Here's how the part is built. I have some questions about the finished solid (model axes, mm). Face numbers are marked on the shaded views. A direction names the side the tool comes from. Round coordinates to 2 decimals unless told otherwise and drop trailing zeros. Loops run counter-clockwise (first coordinate to the right, second up) from the corner with the lowest first, then second, coordinate; pieces in that order, holes last. Notation, with made-up numbers: (-24, 4) - (-18, 4) arc R34 cw to (-18, 38) - close; hole circle Ø4 at (42.5, 9.25). An arc over 180 degrees is marked (long way). Answer as a JSON object with one key per item and string values. Group by question number.
1) I want a section at C-C, the plane y = 7.75. Please give me the cut outline in (x, z), then the cut area to 3 significant figures.
2) I want a section at D-D, the plane z = 8. Please give me the cut outline in (x, y), then the cut area to 3 significant figures.
3) I want a section at B-B, the plane x = -3.5. Please give me the cut outline in (y, z).
4) Which directions (+Z, -Z, +X, -X, +Y, -Y) give clear straight access to the entire face, cutting with the end or side of a thin tool? Please do the marked faces 1, 2 and 3.
5) Will these pins go through, and if not, where does the flat tip stop? P1, Ø1.8, axis at x = 0, y = 0.5, coming from the +Z side; P2, Ø12, axis at y = -7, z = 26.5, coming from the +X side; P3, Ø0.9, axis at y = 7.5, z = 27, coming from the -X side.
6) If we mould it in two halves opening along Y, with no side actions, what happens to the marked faces 4, 5 and 6? For each: pulls with the +Y half, pulls with the -Y half, needs draft (parallel to the pull), parting line crosses it, or undercut.
7) If I drill on line 1 along Y through (x, z) = (0, 34.8); line 2 along Y through (x, z) = (0, 8); line 3 along Z through (x, y) = (2.25, -3.5), over which ranges is the centre line in solid material (lowest first)? Write a range as [from, to].
8) I want a section at A-A, the plane y = 0. Please give me the cut outline in (x, z), then the cut area to 3 significant figures.
from build123d import *
from build123d.topology import SkipClean

# Parameters (mm, degrees)
SKETCH_1_R           = 8.5
EXTRUDE_1_DEPTH      = 35
SKETCH_3_W           = 4
SKETCH_3_H           = 4
CUT_EXTRUDE_1_DEPTH  = 14
EXTRUDE_2_REACH      = 41.016
EXTRUDE_2_END_RADIUS = 8.5
EXTRUDE_3_REACH      = 41.016
EXTRUDE_3_END_RADIUS = 8.5
SKETCH_6_R           = 10
SKETCH_6_R_2         = 8.5
EXTRUDE_4_DEPTH      = 7
SKETCH_7_R           = 8.5
EXTRUDE_5_DEPTH      = 3
EXTRUDE_6_REACH      = 44.617
EXTRUDE_6_END_RADIUS = 8.5
CUT_EXTRUDE_2_DEPTH  = 43.617484675
FILLET_1_R           = 2
CUT_EXTRUDE_START    = -3
SKETCH_10_R          = 10
SKETCH_10_R_2        = 8.5
CUT_EXTRUDE_3_DEPTH  = 3
SKETCH_11_R          = 8.5
EXTRUDE_7_DEPTH      = 1
SKETCH_12_R          = 1
CUT_EXTRUDE_4_DEPTH  = 5
CUT_EXTRUDE_5_DEPTH  = 2
EXTRUDE_START        = 3
SKETCH_14_R          = 1
SKETCH_14_R_2        = 0.85
EXTRUDE_8_DEPTH      = 3
FILLET_2_R           = 0.2
SKETCH_15_W          = 8
SKETCH_15_H          = 8
CUT_EXTRUDE_6_DEPTH  = 6


with BuildPart() as part:
    # 草图1 → 凸台-拉伸1 (new body)
    with BuildSketch(Plane.XY):
        Circle(SKETCH_1_R)
    extrude(amount=EXTRUDE_1_DEPTH)

    # 草图3 → 切除-拉伸1 (cut)
    with BuildSketch(Plane.XY.offset(35)):
        with Locations((0, 8.5)):
            Rectangle(SKETCH_3_W, SKETCH_3_H)
    extrude(amount=-CUT_EXTRUDE_1_DEPTH, mode=Mode.SUBTRACT)

    # 凸台-拉伸2: up to this cylinder (the profile starts inside it)
    with SkipClean():  # the faces are left unmerged after this step: merging them gives an invalid solid
        extrude_2_end = Plane(origin=(0, 0, 21.446736), z_dir=(0, 0, -1)) * Cylinder(EXTRUDE_2_END_RADIUS, 100.032, mode=Mode.PRIVATE)
        # 草图4 → 凸台-拉伸2 (add, up to the surface)
        with BuildSketch(Plane(origin=(0, 6.5, 0), x_dir=(1, 0, 0), z_dir=(0, 1, 0)), mode=Mode.PRIVATE) as extrude_2_sk1:
            with BuildLine():
                Line((2, -21), (0, -21))
                ThreePointArc((0, -21), (1.414213562, -21.585786438), (2, -23))
                Line((2, -23), (2, -21))
            make_face()
        extrude_2_tool1 = extrude(extrude_2_sk1.sketch, amount=EXTRUDE_2_REACH, mode=Mode.PRIVATE) & extrude_2_end
        add(extrude_2_tool1.solids().sort_by_distance((1.553264, 6.5, 21.446736))[0])
        # 草图4 → 凸台-拉伸2 (add, up to the surface)
        with BuildSketch(Plane(origin=(0, 6.5, 0), x_dir=(1, 0, 0), z_dir=(0, 1, 0)), mode=Mode.PRIVATE) as extrude_2_sk2:
            with BuildLine():
                Line((-2, -21), (-2, -23))
                ThreePointArc((-2, -23), (-1.414213562, -21.585786438), (0, -21))
                Line((0, -21), (-2, -21))
            make_face()
        extrude_2_tool2 = extrude(extrude_2_sk2.sketch, amount=EXTRUDE_2_REACH, mode=Mode.PRIVATE) & extrude_2_end
        add(extrude_2_tool2.solids().sort_by_distance((-1.553264, 6.5, 21.446736))[0])

    # 凸台-拉伸3: up to this cylinder (the profile starts inside it)
    with SkipClean():  # the faces are left unmerged after this step: merging them gives an invalid solid
        extrude_3_end = Plane(origin=(0, 0, 32.762904), z_dir=(0, 0, -1)) * Cylinder(EXTRUDE_3_END_RADIUS, 100.032, mode=Mode.PRIVATE)
        # 草图5 → 凸台-拉伸3 (add, up to the surface)
        with BuildSketch(Plane(origin=(0, 6.5, 0), x_dir=(1, 0, 0), z_dir=(0, 1, 0)), mode=Mode.PRIVATE) as extrude_3_sk1:
            with BuildLine():
                Line((-2, -29), (-2, -35))
                Line((-2, -35), (2, -35))
                Line((2, -35), (2, -29))
                ThreePointArc((2, -29), (0, -31), (-2, -29))
            make_face()
        extrude_3_tool1 = extrude(extrude_3_sk1.sketch, amount=EXTRUDE_3_REACH, mode=Mode.PRIVATE) & extrude_3_end
        add(extrude_3_tool1.solids().sort_by_distance((0, 6.5, 32.762904))[0])

    # 草图6 → 凸台-拉伸4 (add)
    with BuildSketch(Plane(origin=(0, 0, 0), x_dir=(-1, 0, 0), z_dir=(0, 0, -1))):
        Circle(SKETCH_6_R)
        Circle(SKETCH_6_R_2, mode=Mode.SUBTRACT)
    extrude(amount=-EXTRUDE_4_DEPTH)

    # 草图7 → 凸台-拉伸5 (add)
    with SkipClean():  # the faces are left unmerged after this step: merging them gives an invalid solid
        with BuildSketch(Plane.XY.offset(35)):
            with Locations(Location((0, 0, 0), (0, 0, 180))):
                Circle(SKETCH_7_R)
        extrude(amount=EXTRUDE_5_DEPTH)

    # 凸台-拉伸6: up to this cylinder (the profile starts inside it)
    with SkipClean():  # the faces are left unmerged after this step: merging them gives an invalid solid
        extrude_6_end = Plane(origin=(0, 0, 22.258337), z_dir=(0, 0, -1)) * Cylinder(EXTRUDE_6_END_RADIUS, 107.234, mode=Mode.PRIVATE)
        # 草图8 → 凸台-拉伸6 (add, up to the surface)
        with BuildSketch(Plane(origin=(0, 6.5, 0), x_dir=(1, 0, 0), z_dir=(0, 1, 0)), mode=Mode.PRIVATE) as extrude_6_sk1:
            with BuildLine():
                Line((-2, -23), (-2, -23.2))
                Line((-2, -23.2), (2, -23.2))
                Line((2, -23.2), (2, -23))
                ThreePointArc((2, -23), (0, -21), (-2, -23))
            make_face()
        extrude_6_tool1 = extrude(extrude_6_sk1.sketch, amount=EXTRUDE_6_REACH, mode=Mode.PRIVATE) & extrude_6_end
        add(extrude_6_tool1.solids().sort_by_distance((0, 6.5, 22.258337))[0])

    # 草图9 → 切除-拉伸2 (cut, through all)
    with SkipClean():  # the faces are left unmerged after this step: merging them gives an invalid solid
        with BuildSketch(Plane(origin=(0, 6.5, 0), x_dir=(1, 0, 0), z_dir=(0, 1, 0))):
            with BuildLine():
                Line((-2, -29), (-2, -29.5))
                Line((-2, -29.5), (-2, -31.5))
                ThreePointArc((-2, -31.5), (0, -33.5), (2, -31.5))
                Line((2, -31.5), (2, -29.5))
                Line((2, -29.5), (2, -29))
                Line((2, -29), (-2, -29))
            make_face()
        extrude(amount=CUT_EXTRUDE_2_DEPTH, mode=Mode.SUBTRACT)

    # 圆角1
    # the kernel refuses this fillet: 2 mm, written as the material it adds along each edge
    with BuildSketch(Plane(origin=(-2, 1.5, 23.2), x_dir=(0, 0, 1), z_dir=(0, 1, 0))) as fillet_1_piece_1_section:
        with BuildLine():
            CenterArc((FILLET_1_R, FILLET_1_R), FILLET_1_R, 180, 90)
            Line((0, FILLET_1_R), (0, 0))
            Line((0, 0), (FILLET_1_R, 0))
        make_face()
    fillet_1_piece_1 = extrude(amount=11.761355821, mode=Mode.PRIVATE)
    fillet_1_piece_1 = fillet_1_piece_1 & Plane(origin=(0, 0, 23.652790229), x_dir=(1, 0, 0), z_dir=(0, 0, -1)) * Cylinder(8.5, 32, mode=Mode.PRIVATE)
    add(fillet_1_piece_1)
    with BuildSketch(Plane(origin=(2, 1.5, 23.2), x_dir=(0, 0, 1), z_dir=(0, 1, 0))) as fillet_1_piece_2_section:
        with BuildLine():
            CenterArc((FILLET_1_R, -FILLET_1_R), FILLET_1_R, 90, 90)
            Line((0, -FILLET_1_R), (0, 0))
            Line((0, 0), (FILLET_1_R, 0))
        make_face()
    fillet_1_piece_2 = extrude(amount=11.761355821, mode=Mode.PRIVATE)
    fillet_1_piece_2 = fillet_1_piece_2 & Plane(origin=(0, 0, 23.652790229), x_dir=(1, 0, 0), z_dir=(0, 0, -1)) * Cylinder(8.5, 32, mode=Mode.PRIVATE)
    add(fillet_1_piece_2)

    # 草图10 → 切除-拉伸3 (cut)
    with BuildSketch(Plane.XY.offset(7).offset(CUT_EXTRUDE_START)):
        with Locations(Location((0, 0, 0), (0, 0, 180))):
            Circle(SKETCH_10_R)
        Circle(SKETCH_10_R_2, mode=Mode.SUBTRACT)
    extrude(amount=CUT_EXTRUDE_3_DEPTH, mode=Mode.SUBTRACT)

    # 草图11 → 凸台-拉伸7 (add)
    with BuildSketch(Plane.XY.offset(38)):
        Circle(SKETCH_11_R)
    extrude(amount=EXTRUDE_7_DEPTH)

    # 草图12 → 切除-拉伸4 (cut)
    with BuildSketch(Plane.XY.offset(39)):
        Circle(SKETCH_12_R)
    extrude(amount=-CUT_EXTRUDE_4_DEPTH, mode=Mode.SUBTRACT)

    # 草图13 → 切除-拉伸5 (cut)
    with BuildSketch(Plane.XY.offset(39)):
        Polygon((0, 2.1), (-1.818653348, 1.05), (-1.818653348, -1.05), (0, -2.1), (1.818653348, -1.05), (1.818653348, 1.05), align=None)
    extrude(amount=-CUT_EXTRUDE_5_DEPTH, mode=Mode.SUBTRACT)

    # 草图14 → 凸台-拉伸8 (add)
    with BuildSketch(Plane.XY.offset(34).offset(EXTRUDE_START)):
        Circle(SKETCH_14_R)
        Circle(SKETCH_14_R_2, mode=Mode.SUBTRACT)
    extrude(amount=-EXTRUDE_8_DEPTH)

    # 圆角2
    fillet_2_edges = [part.edges().sort_by_distance(p)[0] for p in [
        (-0.85, 0, 37),
    ]]
    fillet(fillet_2_edges, radius=FILLET_2_R)

    # 草图15 → 切除-拉伸6 (cut)
    with BuildSketch(Plane(origin=(0, 0, 0), x_dir=(-1, 0, 0), z_dir=(0, 0, -1))):
        Rectangle(SKETCH_15_W, SKETCH_15_H)
    extrude(amount=-CUT_EXTRUDE_6_DEPTH, mode=Mode.SUBTRACT)


solid = part.part
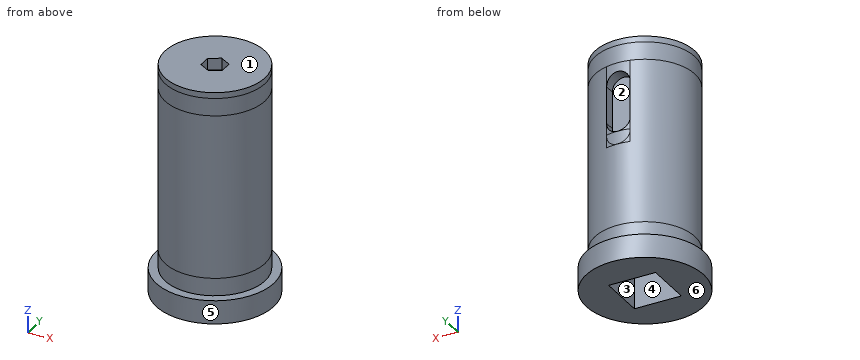
Outcome:
{
 "1": {"outline": "(-6.32, 0) - (6.32, 0) - (6.32, 4) - (3.49, 4) - (3.49, 39) - (-3.49, 39) - (-3.49, 4) - (-6.32, 4) - close; hole (-2, 25.2) arc R2 ccw to (2, 25.2) - (2, 31.5) arc R2 ccw to (-2, 31.5) - close", "area": "257 mm^2"},
 "2": {"outline": "circle Ø17 at (0, 0)", "area": "227 mm^2"},
 "3": {"outline": "(-9.37, 0) - (-4, 0) - (-4, 6) - (4, 6) - (4, 0) - (9.37, 0) - (9.37, 4) - (7.75, 4) - (7.75, 39) - (-7.75, 39) - (-7.75, 4) - (-9.37, 4) - close"},
 "4": {"face 1": "+Z, +X, -X, +Y, -Y", "face 2": "+Y", "face 3": "-Z"},
 "5": {"P1": "z = 37", "P2": "x = 8.44", "P3": "x = -4.75"},
 "6": {"face 4": "undercut", "face 5": "parting line crosses it", "face 6": "needs draft"},
 "7": {"line 1": "[-8.5, -0.85], [0.85, 8.5]", "line 2": "[-8.5, 8.5]", "line 3": "[6, 39]"},
 "8": {"outline": "(-10, 0) - (-4, 0) - (-4, 6) - (4, 6) - (4, 0) - (10, 0) - (10, 4) - (8.5, 4) - (8.5, 39) - (1.82, 39) - (1.82, 37) - (1.05, 37) arc R0.2 ccw to (0.85, 36.8) - (0.85, 34) - (-0.85, 34) - (-0.85, 36.8) arc R0.2 ccw to (-1.05, 37) - (-1.82, 37) - (-1.82, 39) - (-8.5, 39) - (-8.5, 4) - (-10, 4) - close", "area": "615 mm^2"}
}
